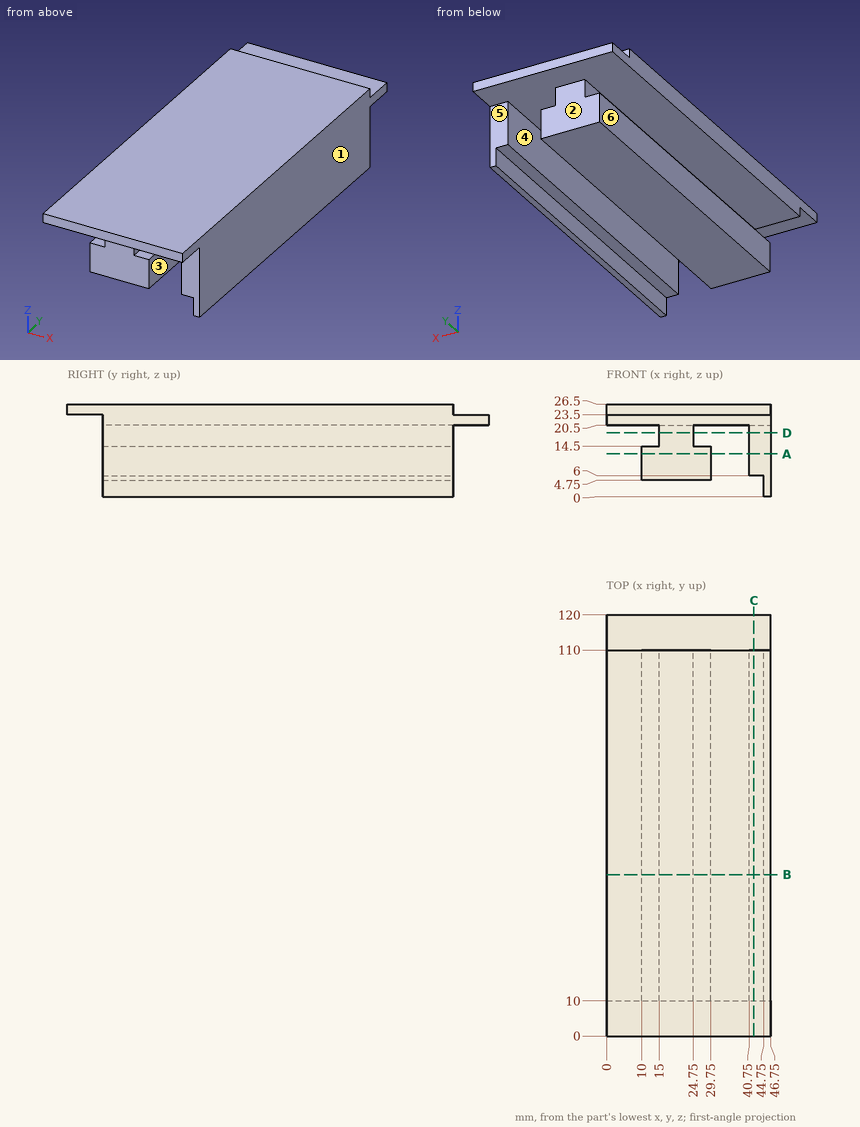
Print and shaded views of the part. All mm, measured from the part's lowest x, y and z. A direction names the side the tool comes from. Round coordinates to 2 decimals unless told otherwise and drop trailing zeros. Order: outer loops, then holes, each group sorted by start corner. A loop starts at its lowest first (then second) coordinate and runs counter-clockwise, first axis right, second up. Notation, with made-up numbers: (82, 89.25) - (133, 89.25) arc R17 ccw to (133, 111.25) - close; hole circle Ø4 at (60, 25.25). An arc over 180 degrees is marked (long way). Use a Markdown table: item, result.
1) Saw through at A-A on z = 12.25. Write the cut outline in (x, y), and give its area (4 significant figures).
Recorded:
| item | result |
|---|---|
| outline | (10, 10) - (29.75, 10) - (29.75, 110) - (10, 110) - close; (40.75, 10) - (46.75, 10) - (46.75, 110) - (40.75, 110) - close |
| area | 2,575 mm² |
2) Flat gauge pins, fed straight in: pin 1 Ø14 at (x, y) = (25, 73.5) entering from -Z; pin 2 Ø5 at (y, z) = (51.5, 7.5) entering from -X; pin 3 Ø10 at (x, z) = (38.5, 13) entering from +Y. Where does each tip first touch, or does it go through?
Recorded:
| item | result |
|---|---|
| pin 1 | stops at z = 4.75 |
| pin 2 | stops at x = 10 |
| pin 3 | stops at y = 110 |
3) Tool access for the marked faces 4, 5 and 6: list every direction of +Z, -Z, +X, -X, +Y, -Y with a clear straight run to the whole face (end or side of a thin tool).
Recorded:
| item | result |
|---|---|
| face 4 | -Z, +Y, -Y |
| face 5 | -Z, +X, -X, +Y |
| face 6 | -Z, -X, +Y, -Y |
4) Wall check: L1, parallel to X at y = 48, z = 5.5; L2, parallel to X at y = 38, z = 10.5; L3, parallel to Z at x = 14, y = 67. Give the ranges that are in metal, low to high.
Recorded:
| item | result |
|---|---|
| L1 | x = 10 to 29.75, 44.75 to 46.75 |
| L2 | x = 10 to 29.75, 40.75 to 46.75 |
| L3 | z = 4.75 to 14.5, 20.5 to 26.5 |
5) Pull direction X, two halves, no side cores. Call the marked faces 1, 2 and 3: pulls with the +X half, pulls with the -X half, needs draft (parallel to the pull), parting line crosses it, or undercut.
Recorded:
| item | result |
|---|---|
| face 1 | pulls with the +X half |
| face 2 | needs draft |
| face 3 | undercut |
6) Saw through at D-D on z = 18.25. Write the cut outline in (x, y).
Recorded:
| item | result |
|---|---|
| outline | (15, 10) - (24.75, 10) - (24.75, 110) - (15, 110) - close; (40.75, 10) - (46.75, 10) - (46.75, 110) - (40.75, 110) - close |
7) Saw through at B-B on y = 46. Write the cut outline in (x, z).
Recorded:
| item | result |
|---|---|
| outline | (0, 20.5) - (15, 20.5) - (15, 14.5) - (10, 14.5) - (10, 4.75) - (29.75, 4.75) - (29.75, 14.5) - (24.75, 14.5) - (24.75, 20.5) - (40.75, 20.5) - (40.75, 6) - (44.75, 6) - (44.75, 0) - (46.75, 0) - (46.75, 26.5) - (0, 26.5) - close |
8) Saw through at C-C on x = 42. Write the cut outline in (y, z), and give its area (3 significant figures).
Recorded:
| item | result |
|---|---|
| outline | (0, 23.5) - (10, 23.5) - (10, 6) - (110, 6) - (110, 20.5) - (120, 20.5) - (120, 23.5) - (110, 23.5) - (110, 26.5) - (0, 26.5) - close |
| area | 2,110 mm² |
